The drawing under review shows one solid part. Ordinate dimensions are in mm from its lowest x, y, z. Give positions to 0.01 mm unless a question says otherwise; leave off trailing zeros. Loops run counter-clockwise (first coordinate to the right, second up) from the corner with the lowest first, then second, coordinate; pieces in that order, holes last.
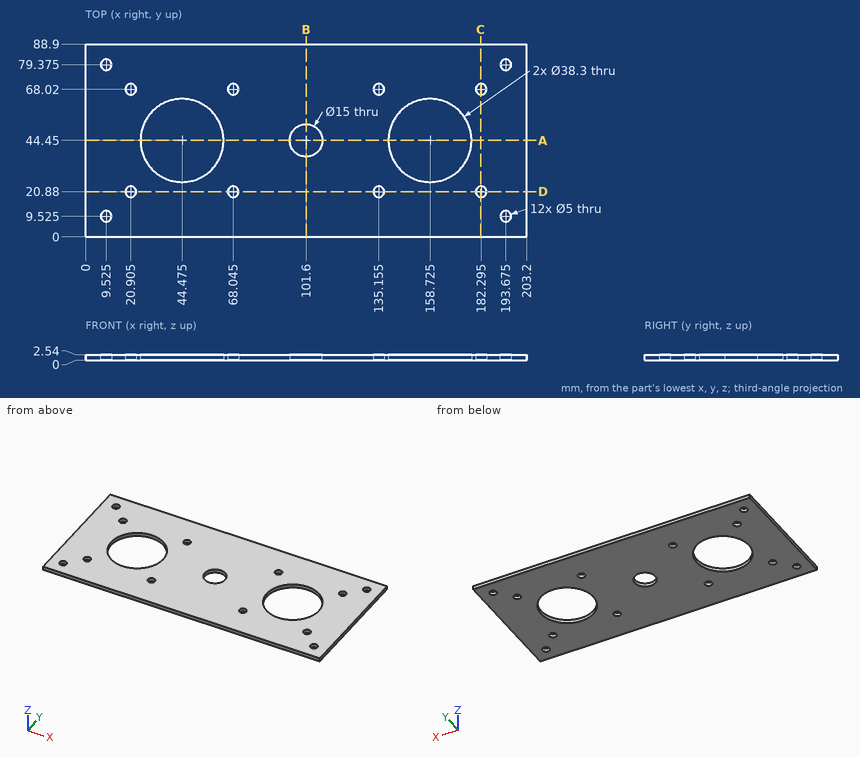
Item 1: Take a section at C-C on x = 182. Give the boundary of the cut face in (y, z).
Answer:
outline: (0, 0) - (18.4, 0) - (18.4, 2.54) - (0, 2.54) - close; (23.36, 0) - (65.54, 0) - (65.54, 2.54) - (23.36, 2.54) - close; (70.5, 0) - (88.9, 0) - (88.9, 2.54) - (70.5, 2.54) - close
Item 2: Clearance check with a flat-ended pin moving along its axis: pin 1 Ø4.5 at (x, y) = (9.525, 79.375) entering from -Z. State where the tip first meets the part, or that it passes through.
Answer:
pin 1: passes through
Item 3: For L1, parallel to X at y = 79, z = 1.05; L2, parallel to Y at x = 157.5, z = 2.15; L3, parallel to Y at x = 183, z = 2.25, list the stretches that pass through material, from the lowest coordinate up.
Answer:
L1: x = 0 to 7.05, 12 to 191.2, 196.15 to 203.2
L2: y = 0 to 25.34, 63.56 to 88.9
L3: y = 0 to 18.48, 23.28 to 65.62, 70.42 to 88.9
Item 4: Take a section at A-A on y = 44.45. Give the boundary of the cut face in (x, z) (3 decimals), and give its area (3 significant figures).
Answer:
outline: (0, 0) - (25.325, 0) - (25.325, 2.54) - (0, 2.54) - close; (63.625, 0) - (94.1, 0) - (94.1, 2.54) - (63.625, 2.54) - close; (109.1, 0) - (139.575, 0) - (139.575, 2.54) - (109.1, 2.54) - close; (177.875, 0) - (203.2, 0) - (203.2, 2.54) - (177.875, 2.54) - close
area: 283 mm2
Item 5: Take a section at D-D on y = 20.88. Give the boundary of the cut face in (x, z) (3 decimals), and give its area (3 significant figures).
Answer:
outline: (0, 0) - (18.405, 0) - (18.405, 2.54) - (0, 2.54) - close; (23.405, 0) - (65.545, 0) - (65.545, 2.54) - (23.405, 2.54) - close; (70.545, 0) - (132.655, 0) - (132.655, 2.54) - (70.545, 2.54) - close; (137.655, 0) - (179.795, 0) - (179.795, 2.54) - (137.655, 2.54) - close; (184.795, 0) - (203.2, 0) - (203.2, 2.54) - (184.795, 2.54) - close
area: 465 mm2
Item 6: Take a section at B-B on x = 101.6. Give the boundary of the cut face in (y, z).
Answer:
outline: (0, 0) - (36.95, 0) - (36.95, 2.54) - (0, 2.54) - close; (51.95, 0) - (88.9, 0) - (88.9, 2.54) - (51.95, 2.54) - close
